Can you work these out from the drawing? Everything is in mm from the part's minimum corner. A direction names the side the tool comes from. Coordinates: 2 decimals unless noted, no trailing zeros. Loops run counter-clockwise (first coordinate to the right, second up) from the corner with the lowest first, then second, coordinate; pieces in that order, holes last. Notation, with made-up numbers: (15, 76.25) -> (34, 76.25) arc R31 ccw to (34, 111.25) -> close; hole circle Ø3 at (7, 73.5). An arc over 180 degrees is marked (long way). Put each result on its own line as item: value. Start each with the question number.
Item 1: If we section it at A-A on x = 34: Please give me the cut outline in (y, z), plus the area to 4 significant figures.
Item 2: If we section it at C-C on z = 124.5: Please give me the cut outline in (x, y).
Item 3: If we section it at B-B on y = 34: Please give me the cut outline in (x, z), plus the area to 3 significant figures.
Item 4: For the marked faces 1, 2 and 3, which set-ups out of +Z, -Z, +X, -X, +Y, -Y let a thin tool reach every point of the face, with its end or its side?
Item 5: Please list where these lines run through material, in increasing order: L1, parallel to Y at x = 34, z = 92.75; L2, parallel to Y at x = 35, z = 45.5 (1 decimal); L3, parallel to Z at x = 30, y = 56. Write a range as from..to.
Item 6: If we section it at D-D on z = 90: State how many separate pieces and enclosed holes the cut face has, plus the area to 4 significant figures.
Item 7: Will these pins go through, and if not, where does the flat tip stop? P1, Ø5, axis at x = 34, y = 12.78, coming from the -Z side; P2, Ø1.3, axis at x = 33.5, y = 13.5, coming from the +Z side; P3, Ø6, axis at y = 57.5, z = 70, coming from the +X side (1 decimal).
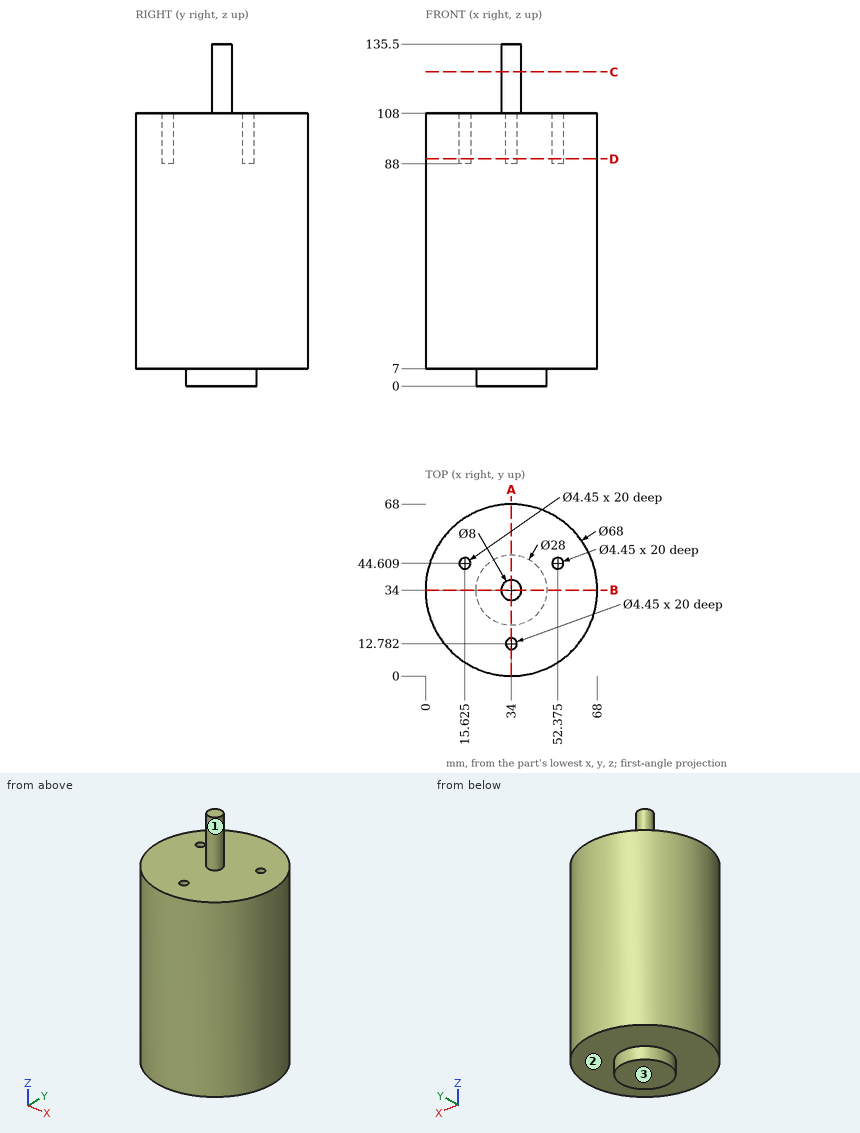
Solutions:
1. outline: (0, 7) -> (20, 7) -> (20, 0) -> (48, 0) -> (48, 7) -> (68, 7) -> (68, 108) -> (38, 108) -> (38, 135.5) -> (30, 135.5) -> (30, 108) -> (15.01, 108) -> (15.01, 88) -> (10.56, 88) -> (10.56, 108) -> (0, 108) -> close
1. area: 7,195 mm^2
2. outline: circle Ø8 at (34, 34)
3. outline: (0, 7) -> (20, 7) -> (20, 0) -> (48, 0) -> (48, 7) -> (68, 7) -> (68, 108) -> (38, 108) -> (38, 135.5) -> (30, 135.5) -> (30, 108) -> (0, 108) -> close
3. area: 7,280 mm^2
4. face 1: +Z
4. face 2: -Z
4. face 3: -Z, +X, -X, +Y, -Y
5. L1: 0..10.56, 15.01..68
5. L2: 0..68
5. L3: 7..108
6. separate pieces: 1
6. enclosed holes: 3
6. area: 3,585 mm^2
7. P1: z = 7
7. P2: z = 88
7. P3: x = 61.1
